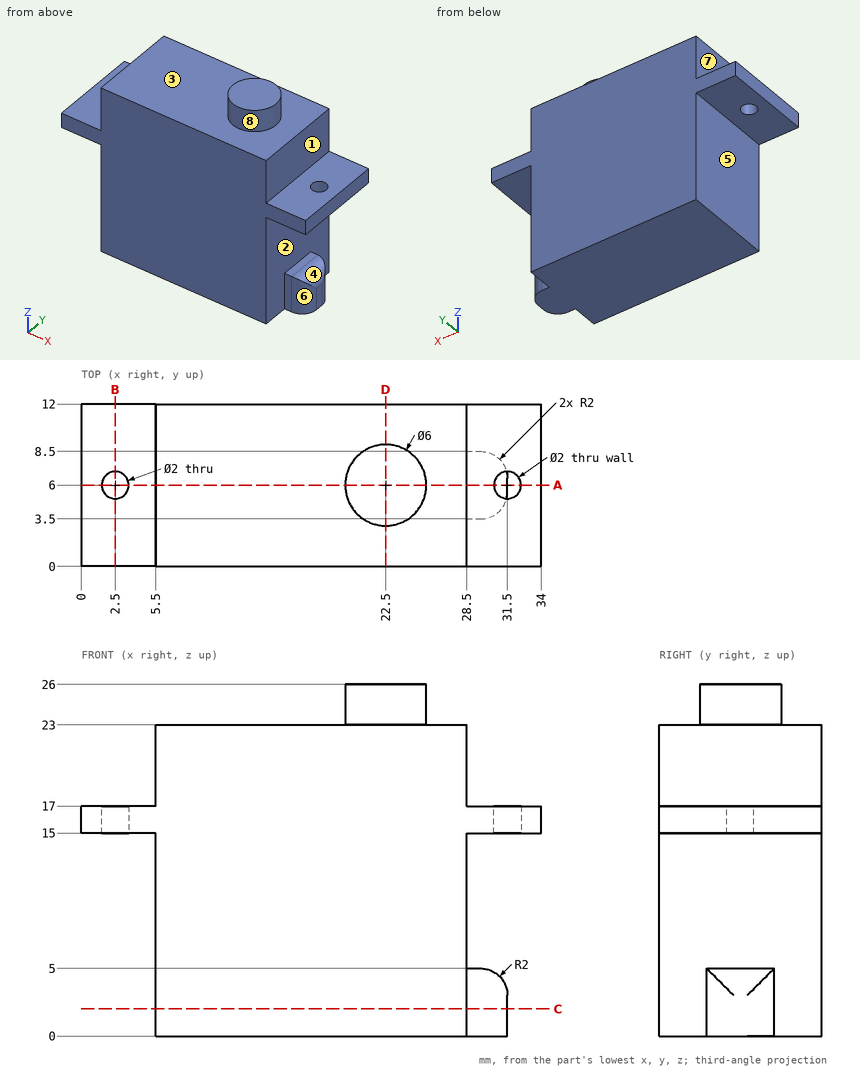
Input: dimensioned drawing with shaded views. Units: mm. Origin: part minimum x, y, z. A direction names the side the tool comes from. Coordinates: 2 decimals unless noted, no trailing zeros. Order: outer loops, then holes, each group sorted by start corner. A loop starts at its lowest first (then second) coordinate and runs counter-clockwise, first axis right, second up. Notation, with made-up numbers: (-21.75, -4) - (4.25, -4) arc R10 cw to (4.25, 1) - close; hole circle Ø11 at (24.5, 12). An arc over 180 degrees is marked (long way). Return JSON: item names as keys, results as strings. Group by question number.
1. Cut plane A-A (y = 6). Output: boundary loops of the cut face in (x, z).
2. Cut plane D-D (x = 22.5). Output: boundary loops of the cut face in (y, z), plus the area to 3 significant figures.
3. Material intervals for line 1 along Y through (x, z) = (2.5, 16.5); line 2 along Z through (x, y) = (19.5, 9.25); line 3 along X through (y, z) = (10, 2.5), sorted ascending. Write a range as [from, to].
4. Cut plane B-B (x = 2.5). Output: boundary loops of the cut face in (y, z).
5. Cut plane C-C (z = 2). Output: boundary loops of the cut face in (x, y), plus the area to 3 significant figures.
6. Pull-direction query (Z, two-part tool) for the marked faces 1, 2 and 3; classes: pulls with the +Z half, pulls with the -Z half, needs draft (parallel to the pull), parting line crosses it, or undercut.
7. Set-up query: the marked faces 4, 5, 6, 7 and 8. Return all of +Z, -Z, +X, -X, +Y, -Y with unobstructed straight access to the full face (end or side cutting, diameter ignored); none if empty.
8. Pin query (flat end, axial travel): pin 1 (6.5 mm diameter, centred on y = 9, z = 21, fed in from -X); pin 2 (5 mm diameter, centred on y = 5.5, z = 20.5, fed in from +X); pin 3 (1.6 mm diameter, centred on x = 4, y = 7.5, fed in from +Z). Return the tip coordinate at first contact, or that it passes through.
Resolved:
{
 "1": {"outline": "(0, 15) - (1.5, 15) - (1.5, 17) - (0, 17) - close; (3.5, 15) - (5.5, 15) - (5.5, 0) - (31.5, 0) - (31.5, 3) arc R2 ccw to (29.5, 5) - (28.5, 5) - (28.5, 15) - (30.5, 15) - (30.5, 17) - (28.5, 17) - (28.5, 23) - (25.5, 23) - (25.5, 26) - (19.5, 26) - (19.5, 23) - (5.5, 23) - (5.5, 17) - (3.5, 17) - close; (32.5, 15) - (34, 15) - (34, 17) - (32.5, 17) - close"},
 "2": {"outline": "(0, 0) - (12, 0) - (12, 23) - (9, 23) - (9, 26) - (3, 26) - (3, 23) - (0, 23) - close", "area": "294 mm²"},
 "3": {"line 1": "y = [0, 5], [7, 12]", "line 2": "z = [0, 23]", "line 3": "x = [5.5, 28.5]"},
 "4": {"outline": "(0, 15) - (5, 15) - (5, 17) - (0, 17) - close; (7, 15) - (12, 15) - (12, 17) - (7, 17) - close"},
 "5": {"outline": "(5.5, 0) - (28.5, 0) - (28.5, 3.5) - (29.5, 3.5) arc R2 ccw to (31.5, 5.5) - (31.5, 6.5) arc R2 ccw to (29.5, 8.5) - (28.5, 8.5) - (28.5, 12) - (5.5, 12) - close", "area": "289 mm²"},
 "6": {"face 1": "needs draft", "face 2": "undercut", "face 3": "pulls with the +Z half"},
 "7": {"face 4": "+X, +Y, -Y", "face 5": "-Z, -X, +Y, -Y", "face 6": "-Z, +X, -Y", "face 7": "+Z, -X, +Y, -Y", "face 8": "+Z"},
 "8": {"pin 1": "stops at x = 5.5", "pin 2": "stops at x = 28.5", "pin 3": "stops at z = 17"}
}
